Verification items for the finished model (mm, model axes). Face numbers are marked on the shaded views. A direction names the side the tool comes from. Coordinates: 2 decimals unless noted, no trailing zeros. Loops run counter-clockwise (first coordinate to the right, second up) from the corner with the lowest first, then second, coordinate; pieces in that order, holes last. Notation, with made-up numbers: (65.25, 71.25) -> (70.25, 71.25) arc R23 cw to (70.25, 83.25) -> close; hole circle Ø7 at (32, 73.5). An arc over 180 degrees is marked (long way). Write item = value, one per line.
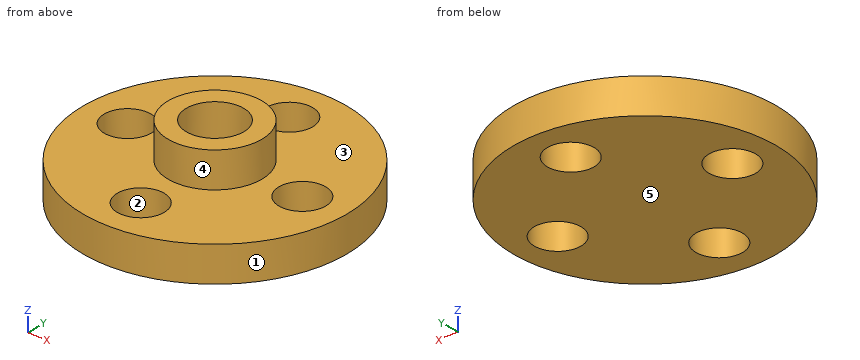
```python
from build123d import *

# Parameters (mm, degrees)
SKIZZE1_R                       = 11.25
AUFSATZ_LINEAR_AUSTRAGEN1_DEPTH = 3
SKIZZE2_R                       = 4
SKIZZE2_R_2                     = 2.45
AUFSATZ_LINEAR_AUSTRAGEN2_DEPTH = 3
SCHNITT_LINEAR_AUSTRAGEN1_REACH = 18.19
SKIZZE3_R                       = 2


with BuildPart() as part:
    # Skizze1 → Aufsatz-Linear austragen1 (new body)
    with BuildSketch(Plane.XY):
        Circle(SKIZZE1_R)
    extrude(amount=-AUFSATZ_LINEAR_AUSTRAGEN1_DEPTH)

    # Skizze2 → Aufsatz-Linear austragen2 (add)
    with BuildSketch(Plane.XY):
        Circle(SKIZZE2_R)
        Circle(SKIZZE2_R_2, mode=Mode.SUBTRACT)
    extrude(amount=AUFSATZ_LINEAR_AUSTRAGEN2_DEPTH)

    # Skizze3 → Schnitt-Linear austragen1 (cut, up to next)
    with BuildSketch(Plane.XY, mode=Mode.PRIVATE) as schnitt_linear_austragen1_sk1:
        with Locations((0, 7.5)):
            Circle(SKIZZE3_R)
    schnitt_linear_austragen1_tool1 = extrude(schnitt_linear_austragen1_sk1.sketch, amount=-SCHNITT_LINEAR_AUSTRAGEN1_REACH, mode=Mode.PRIVATE) & part.part
    # Skizze3 → Schnitt-Linear austragen1 (cut, up to next)
    with BuildSketch(Plane.XY, mode=Mode.PRIVATE) as schnitt_linear_austragen1_sk2:
        with Locations((7.5, 0)):
            Circle(SKIZZE3_R)
    schnitt_linear_austragen1_tool2 = extrude(schnitt_linear_austragen1_sk2.sketch, amount=-SCHNITT_LINEAR_AUSTRAGEN1_REACH, mode=Mode.PRIVATE) & part.part
    # Skizze3 → Schnitt-Linear austragen1 (cut, up to next)
    with BuildSketch(Plane.XY, mode=Mode.PRIVATE) as schnitt_linear_austragen1_sk3:
        with Locations((0, -7.5)):
            Circle(SKIZZE3_R)
    schnitt_linear_austragen1_tool3 = extrude(schnitt_linear_austragen1_sk3.sketch, amount=-SCHNITT_LINEAR_AUSTRAGEN1_REACH, mode=Mode.PRIVATE) & part.part
    # Skizze3 → Schnitt-Linear austragen1 (cut, up to next)
    with BuildSketch(Plane.XY, mode=Mode.PRIVATE) as schnitt_linear_austragen1_sk4:
        with Locations((-7.5, 0)):
            Circle(SKIZZE3_R)
    schnitt_linear_austragen1_tool4 = extrude(schnitt_linear_austragen1_sk4.sketch, amount=-SCHNITT_LINEAR_AUSTRAGEN1_REACH, mode=Mode.PRIVATE) & part.part
    add(schnitt_linear_austragen1_tool1.solids().sort_by_distance((0, 7.5, 0))[0], mode=Mode.SUBTRACT)
    add(schnitt_linear_austragen1_tool2.solids().sort_by_distance((7.5, 0, 0))[0], mode=Mode.SUBTRACT)
    add(schnitt_linear_austragen1_tool3.solids().sort_by_distance((0, -7.5, 0))[0], mode=Mode.SUBTRACT)
    add(schnitt_linear_austragen1_tool4.solids().sort_by_distance((-7.5, 0, 0))[0], mode=Mode.SUBTRACT)


solid = part.part
```
1) Release check for a two-part mould opening along Y. For the marked faces 1, 2 and 3 record: pulls with the +Y half, pulls with the -Y half, needs draft (parallel to the pull), parting line crosses it, or undercut.
Ans:
face_1 = parting line crosses it
face_2 = undercut
face_3 = needs draft
2) Tool access check on the marked faces 4 and 5. Record the directions out of +Z, -Z, +X, -X, +Y, -Y that give a thin tool (end or side, any length) a straight path to the whole face; none if there is none.
Ans:
face_4 = +Z
face_5 = -Z, +X, -X, +Y, -Y
3) Material ranges on line 1 (Y direction, x = 0, z = -1); line 2 (Z direction, x = -2, y = -6.75); line 3 (Y direction, x = 0, z = 0.7), recorded low to high.
Ans:
line_1 = -11.25 to -9.5, -5.5 to 5.5, 9.5 to 11.25
line_2 = -3 to 0
line_3 = -4 to -2.45, 2.45 to 4
4) Sectioned sample at C-C, the plane x = -7.5. Record the cut outline in (y, z), plus the area to 3 significant figures.
Ans:
outline = (-8.39, -3) -> (-2, -3) -> (-2, 0) -> (-8.39, 0) -> close; (2, -3) -> (8.39, -3) -> (8.39, 0) -> (2, 0) -> close
area = 38.3 mm2
5) Sectioned sample at A-A, the plane y = 0. Record the cut outline in (x, z).
Ans:
outline = (-11.25, -3) -> (-9.5, -3) -> (-9.5, 0) -> (-11.25, 0) -> close; (-5.5, -3) -> (5.5, -3) -> (5.5, 0) -> (4, 0) -> (4, 3) -> (2.45, 3) -> (2.45, 0) -> (-2.45, 0) -> (-2.45, 3) -> (-4, 3) -> (-4, 0) -> (-5.5, 0) -> close; (9.5, -3) -> (11.25, -3) -> (11.25, 0) -> (9.5, 0) -> close
6) Depth check by flat-ended pin: pin 1 Ø2.5 at (x, y) = (-1, 0) entering from +Z; pin 2 Ø1.5 at (x, z) = (-9, -0.5) entering from +Y; pin 3 Ø2.5 at (x, y) = (7.5, 0) entering from -Z; pin 4 Ø3 at (y, z) = (-4.5, 0.5) entering from -X. Enter the tip coordinate at first touch or a pass-through.
Ans:
pin_1 = 0
pin_2 = 7.65
pin_3 = through
pin_4 = -10.82
7) Sectioned sample at B-B, the plane z = -0.9. Record the cut outline in (x, y), plus the area to 3 significant figures.
Ans:
outline = circle Ø22.5 at (0, 0); hole circle Ø4 at (-7.5, 0); hole circle Ø4 at (0, -7.5); hole circle Ø4 at (0, 7.5); hole circle Ø4 at (7.5, 0)
area = 347 mm2
